```python
from build123d import *

# Parameters (mm, degrees)
F4_D           = 4.2
F4_CBORE_D     = 8.25
F4_CBORE_DEPTH = 4
F5_D           = 6.3
F5_CBORE_D     = 11.25
F5_CBORE_DEPTH = 6
F6_SIZE        = 2
F7_SIZE        = 0.5


with BuildPart() as f1:
    # F0 (on Front) → F1 (revolve)
    with BuildSketch(Plane.XZ):
        Polygon((-4.6182575495, 105), (-4.6182575495, 80), (-6.6182575495, 80), (-6.6182575495, 74), (-4.6182575495, 74), (-4.6182575495, 40), (8.0817424505, 40), (8.0817424505, 52.5), (7.5817424505, 52.5), (7.5817424505, 105), align=None)
    revolve(axis=Axis((-22.0904547029, 0, 0), (-1, 0, 0)))

    # F4 (through all)
    with Locations(Plane(origin=(-4.6182575495, 0, 0), x_dir=(0, -1, 0), z_dir=(-1, 0, 0))):
        with Locations((0, 46), (23, 39.8371685741), (39.8371685741, 23), (46, 0), (39.8371685741, -23), (23, -39.8371685741), (0, -46), (-23, -39.8371685741), (-46, 0), (-39.8371685741, -23), (-39.8371685741, 23), (-23, 39.8371685741)):
            CounterBoreHole(F4_D / 2, F4_CBORE_D / 2, F4_CBORE_DEPTH)

    # F5 (through all)
    with Locations(Plane.YZ.offset(7.5817424505)):
        with Locations((0, 90), (45, 77.9422863406), (77.9422863406, 45), (90, 0), (77.9422863406, -45), (45, -77.9422863406), (0, -90), (-45, -77.9422863406), (-77.9422863406, -45), (-90, 0), (-77.9422863406, 45), (-45, 77.9422863406)):
            CounterBoreHole(F5_D / 2, F5_CBORE_D / 2, F5_CBORE_DEPTH)

    # F6
    f6_edges = [f1.edges().sort_by_distance(p)[0] for p in [
        (7.581742, 0, -105),
    ]]
    chamfer(f6_edges, length=F6_SIZE)

    # F7
    f7_edges = [f1.edges().sort_by_distance(p)[0] for p in [
        (-6.618258, 0, -80),
        (-6.618258, 0, -74),
        (8.081742, 0, -40),
        (-4.618258, 0, -40),
    ]]
    chamfer(f7_edges, length=F7_SIZE)


solid = f1.part
```
Geometry check sheet. Reference: the model listing, model coordinates, mm. A direction names the side the tool comes from. Give positions to 0.01 mm unless a question says otherwise; leave off trailing zeros. Use one line per item in the form item = value.
Item 1: Scan lines: line 1 (Z direction, x = 5, y = 74); line 2 (Z direction, x = 3.5, y = 23); line 3 (Z direction, x = 5.5, y = 46). Record each from-to range of solid material in increasing order.
Results list:
line_1 = -74.49 to -49.01, -40.99 to 40.99, 49.01 to 74.49
line_2 = -102.45 to -41.94, -37.74 to -32.73, 32.73 to 37.74, 41.94 to 102.45
line_3 = -94.39 to -83.48, -72.41 to -2.1, 2.1 to 72.41, 83.48 to 94.39
Item 2: Mould release check, pull along Y, two halves, no side actions. Record for faces 4 (the cylindrical face through (4.624, -0.732, 95.577)), 5 (the cylindrical face through (-2.65, -42.05, 26.48)), 6 (the cylindrical face through (7.828, 15.77, 50.076)): released by +Y, released by -Y, zero draft, split by the parting line, or undercut.
Results list:
face_4 = undercut
face_5 = undercut
face_6 = split by the parting line
Item 3: Access from +Z, -Z, +X, -X, +Y, -Y to the whole of each face (thin tool, end or side, straight path). Record for faces 1 (the flat face through (1.582, 80.4, 42.6)), 2 (the flat face through (-0.618, 42, 24)), 3 (the cylindrical face through (-1.562, -74.795, 45.138)).
Results list:
face_1 = +X
face_2 = -X
face_3 = +X, -X
Item 4: Depth check by flat-ended pin: pin 1 Ø5.5 at (y, z) = (-2.5, 92) entering from +X; pin 2 Ø9.5 at (y, z) = (46, 0) entering from -X; pin 3 Ø7 at (y, z) = (90, 0) entering from +X; pin 4 Ø5.5 at (y, z) = (-77.94, 45) entering from +X. Enter the tip coordinate at first touch or a pass-through.
Results list:
pin_1 = 7.58
pin_2 = -4.62
pin_3 = 1.58
pin_4 = through
